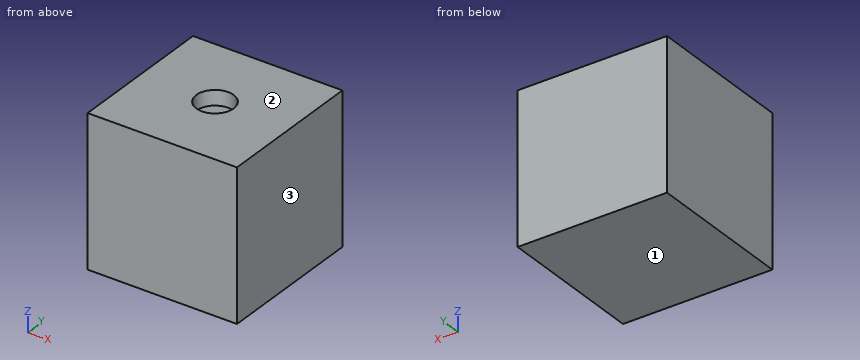
from build123d import *

# Parameters (mm, degrees)
ESQUISSE1_W             = 20
ESQUISSE1_H             = 20
BOSS_EXTRU_1_DEPTH      = 20
ESQUISSE2_R             = 2.5
ENL_V_MAT_EXTRU_1_DEPTH = 2


with BuildPart() as part:
    # Esquisse1 → Boss.-Extru.1 (new body)
    with BuildSketch(Plane.XY):
        with Locations((10, 10)):
            Rectangle(ESQUISSE1_W, ESQUISSE1_H)
    extrude(amount=-BOSS_EXTRU_1_DEPTH)

    # Esquisse2 → Enlèv. mat.-Extru.1 (cut)
    with BuildSketch(Plane.XY):
        with Locations((10, 10)):
            Circle(ESQUISSE2_R)
    extrude(amount=-ENL_V_MAT_EXTRU_1_DEPTH, mode=Mode.SUBTRACT)


solid = part.part
Can you work these out from the model? Positions are in its coordinate system, mm. Face numbers are marked on the shaded views. Round coordinates to 2 decimals unless told otherwise and drop trailing zeros. Order: outer loops, then holes, each group sorted by start corner. A loop starts at its lowest first (then second) coordinate and runs counter-clockwise, first axis right, second up. Notation, with made-up numbers: (84, 10.25) -> (117, 10.25) arc R20 ccw to (117, 39.25) -> close; hole circle Ø4 at (18, 49). An arc over 180 degrees is marked (long way). Write each question's results on one line, items separated by ' | '. Start each with the question number.
Item 1: Thinking about a two-plate mould opening in Z: for the marked faces 1, 2 and 3, which applies, +Z half, -Z half, draft (parallel to the pull), parting line (faces both ways), or undercut?
Item 2: If we section it at A-A, the plane x = 10: Write out the boundary of the cut face in (y, z).
Item 3: Please list where this line runs through material, in increasing order: L1, parallel to Y at x = 10, z = -1.1.
Item 4: Will this pin go through, and if not, where does the flat tip stop? pin 1 (1.5 mm diameter, centred on x = 9, y = 11, fed in from +Z).
Results:
1) face 1: -Z half | face 2: +Z half | face 3: draft
2) outline: (0, -20) -> (20, -20) -> (20, 0) -> (12.5, 0) -> (12.5, -2) -> (7.5, -2) -> (7.5, 0) -> (0, 0) -> close
3) L1: y = 0 to 7.5, 12.5 to 20
4) pin 1: stops at z = -2
